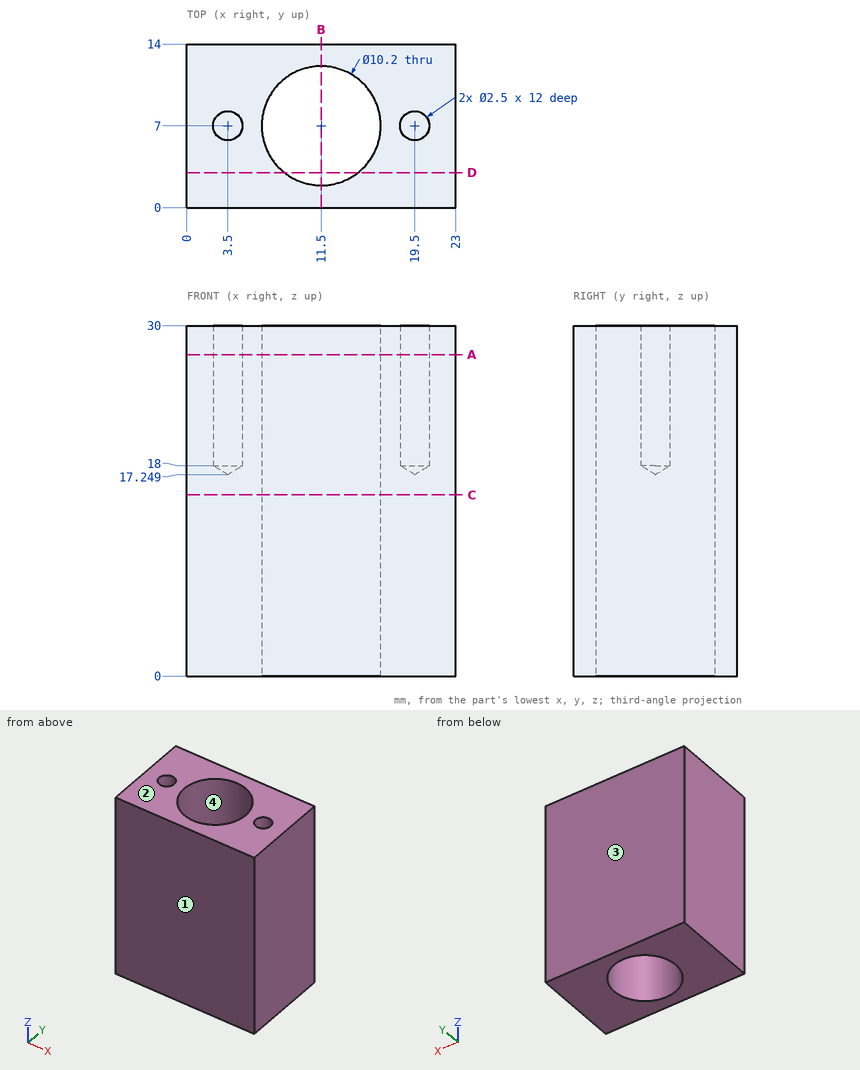
Study the drawing (mm; zero at the part's minimum x, y, z) and answer. Coordinates: 2 decimals unless noted, no trailing zeros. Loops run counter-clockwise (first coordinate to the right, second up) from the corner with the lowest first, then second, coordinate; pieces in that order, holes last. Notation, with made-up numbers: (43.5, 67.25) -> (58.5, 67.25) arc R20 cw to (58.5, 88.25) -> close; hole circle Ø4 at (18, 31). An arc over 180 degrees is marked (long way). Write each question's results on one line, items separated by ' | '. Start each with the question number.
1) Consider line 1 along Y through (x, z) = (11.5, 18); line 2 along Y through (x, z) = (3.5, 27.25); line 3 along X through (y, z) = (3.75, 5). Determine where each line is inside the solid, lowest interval first.
2) Find section D-D on y = 3. Determine the outline of the cut face in (x, z), then the cut area to 3 significant figures.
3) Find section A-A on z = 27.5. Determine the outline of the cut face in (x, y), then the cut area to 3 significant figures.
4) Find section B-B on x = 11.5. Determine the outline of the cut face in (y, z).
5) Find section C-C on z = 15.5. Determine the outline of the cut face in (x, y).
6) The mould has two halves that part along Y. Classify the marked faces 1, 2, 3 and 4: pulls with the +Y half, pulls with the -Y half, needs draft (parallel to the pull), parting line crosses it, or undercut.
Response values:
1) line 1: y = 0 to 1.9, 12.1 to 14 | line 2: y = 0 to 5.75, 8.25 to 14 | line 3: x = 0 to 7.57, 15.43 to 23
2) outline: (0, 0) -> (8.34, 0) -> (8.34, 30) -> (0, 30) -> close; (14.66, 0) -> (23, 0) -> (23, 30) -> (14.66, 30) -> close | area: 500 mm^2
3) outline: (0, 0) -> (23, 0) -> (23, 14) -> (0, 14) -> close; hole circle Ø2.5 at (3.5, 7); hole circle Ø10.2 at (11.5, 7); hole circle Ø2.5 at (19.5, 7) | area: 230 mm^2
4) outline: (0, 0) -> (1.9, 0) -> (1.9, 30) -> (0, 30) -> close; (12.1, 0) -> (14, 0) -> (14, 30) -> (12.1, 30) -> close
5) outline: (0, 0) -> (23, 0) -> (23, 14) -> (0, 14) -> close; hole circle Ø10.2 at (11.5, 7)
6) face 1: pulls with the -Y half | face 2: needs draft | face 3: pulls with the +Y half | face 4: undercut
